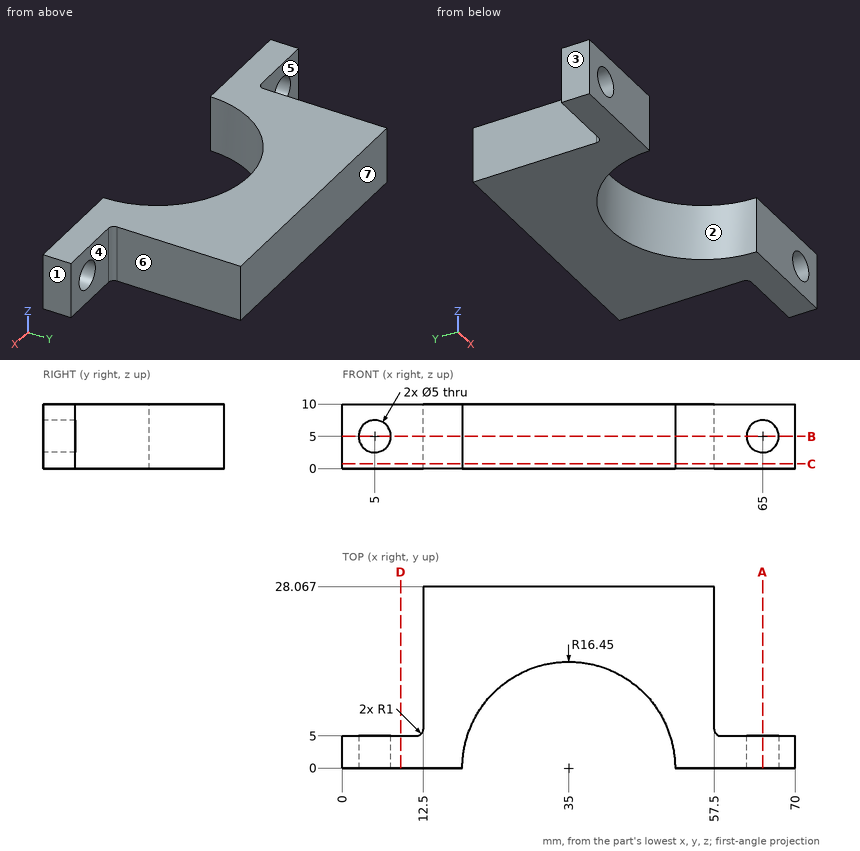
Source: three-view drawing plus pictorial views. Frame: mm from the lowest corner of the part. A direction names the side the tool comes from. Round coordinates to 2 decimals unless told otherwise and drop trailing zeros. Loops run counter-clockwise (first coordinate to the right, second up) from the corner with the lowest first, then second, coordinate; pieces in that order, holes last. Notation, with made-up numbers: (12.5, 70) - (62.5, 70) arc R18 ccw to (62.5, 76) - close; hole circle Ø9 at (27, 42.25). An arc over 180 degrees is marked (long way). Write each question's results on one line, items separated by ' | '. Start each with the question number.
1) Access query for the marked faces 5, 6 and 7. Directions: +Z, -Z, +X, -X, +Y, -Y. A direction counts if a zero-diameter tool reaches every point of the face in a straight line with its end or side. Return the directions, or none.
2) Mould query, pull axis X, two halves, no side actions, for the marked faces 1, 2, 3 and 4. Classes: released by +X, released by -X, zero draft, split by the parting line, or undercut.
3) First-contact query: P1, Ø2, axis at y = 21, z = 8, coming from the +X side; P2, Ø3, axis at x = 65, z = 5, coming from the +Y side; P3, Ø4, axis at y = 9, z = 7, coming from the -X side; P4, Ø2, axis at x = 55.5, y = 22.5, coming from the -Z side. Flat tips, straight axial feed; report the tip coordinate or a pass-through.
4) Cut plane A-A on x = 65. Return loops of the section in (y, z), then the cut area to 3 significant figures.
5) Line query: probe 1 along Z at (x, y) = (65, 3.9); probe 2 along Y at (x, z) = (63.5, 7.5); probe 3 along X at (y, z) = (24.75, 3). Output: solid intervals per line, ascending. Write a range as [from, to].
6) Cut plane C-C on z = 0.75. Return loops of the section in (x, y), then the cut area to 3 significant figures.
7) Cut plane B-B on z = 5. Return loops of the section in (x, y), then the cut area to 3 significant figures.
8) Cut plane D-D on x = 9. Return loops of the section in (y, z), then the cut area to 3 significant figures.
Verdict:
1) face 5: +Z, -Z, -X, +Y | face 6: +Z, -Z, +X, +Y | face 7: +Z, -Z, +X, -X, +Y
2) face 1: released by +X | face 2: undercut | face 3: released by -X | face 4: zero draft
3) P1: stops at x = 57.5 | P2: passes through | P3: stops at x = 12.5 | P4: stops at z = 0
4) outline: (0, 0) - (5, 0) - (5, 2.5) - (0, 2.5) - close; (0, 7.5) - (5, 7.5) - (5, 10) - (0, 10) - close | area: 25.0 mm2
5) probe 1: z = [0, 2.5], [7.5, 10] | probe 2: y = [0, 5] | probe 3: x = [12.5, 57.5]
6) outline: (0, 0) - (18.55, 0) arc R16.45 cw to (51.45, 0) - (70, 0) - (70, 5) - (58.5, 5) arc R1 cw to (57.5, 6) - (57.5, 28.07) - (12.5, 28.07) - (12.5, 6) arc R1 cw to (11.5, 5) - (0, 5) - close | area: 963 mm2
7) outline: (0, 0) - (2.5, 0) - (2.5, 5) - (0, 5) - close; (7.5, 0) - (18.55, 0) arc R16.45 cw to (51.45, 0) - (62.5, 0) - (62.5, 5) - (58.5, 5) arc R1 cw to (57.5, 6) - (57.5, 28.07) - (12.5, 28.07) - (12.5, 6) arc R1 cw to (11.5, 5) - (7.5, 5) - close; (67.5, 0) - (70, 0) - (70, 5) - (67.5, 5) - close | area: 913 mm2
8) outline: (0, 0) - (5, 0) - (5, 10) - (0, 10) - close | area: 50.0 mm2
